```python
from build123d import *

# Parameters (mm, degrees)
BASENUTSKE_R       = 4
BASENUT_DEPTH      = 4
SKETCH6_OUTSIDE_W  = 38.384
SKETCH6_OUTSIDE_H  = 36.372
SKETCH6_OUTSIDE_R  = 6.175
CUT_EXTRUDE2_DEPTH = 5
CUT_EXTRUDE2_TAPER = 60


with BuildPart() as part:
    # BaseNutSke → BaseNut (new body)
    with BuildSketch(Plane.XY):
        Polygon((3.75277675, -6.5), (-3.75277675, -6.5), (-7.505553499, 0), (-3.75277675, 6.5), (3.75277675, 6.5), (7.505553499, 0), align=None)
        Circle(BASENUTSKE_R, mode=Mode.SUBTRACT)
    extrude(amount=-BASENUT_DEPTH)

    # Sketch6 outside → Cut-Extrude2 (cut, through all)
    with BuildSketch(Plane(origin=(0, 0, -4), x_dir=(-1, 0, 0), z_dir=(0, 0, -1))):
        Rectangle(SKETCH6_OUTSIDE_W, SKETCH6_OUTSIDE_H)
        Circle(SKETCH6_OUTSIDE_R, mode=Mode.SUBTRACT)
    cut_extrude2 = extrude(amount=-CUT_EXTRUDE2_DEPTH, taper=CUT_EXTRUDE2_TAPER, mode=Mode.SUBTRACT)

    # Mirror1: Cut-Extrude2 across plane
    add(cut_extrude2.mirror(Plane(origin=(0, 0, -2), x_dir=(1, 0, 0), z_dir=(0, 0, -1))), mode=Mode.SUBTRACT)


solid = part.part
```
Here's how the part is built. I have some questions about the finished solid (model axes, mm). Give positions to 0.01 mm unless a question says otherwise; leave off trailing zeros. Order: outer loops, then holes, each group sorted by start corner. A loop starts at its lowest first (then second) coordinate and runs counter-clockwise, first axis right, second up. Notation, with made-up numbers: (42.5, 40.5) -> (62.5, 40.5) arc R15 ccw to (62.5, 67.5) -> close; hole circle Ø10 at (-16, 57.25). An arc over 180 degrees is marked (long way). Use CSV: the item, a comma, the result in double quotes. Start each with the question number.
Item 1: Suppose I cut it at C-C (z = -3.6). List the corners of the cut face in (x, y) for me.
Item 2: Thinking about a two-plate mould opening in X: for faces 1 (the flat face through (0, 6.5, -2)), 2 (the flat face through (5.6, 3.3, -2)), 3 (the flat face through (-5.66, 3.2, -1.97)), 4 (the cylindrical face through (-0.867, -3.905, -1.972)), which applies, pulls with the +X half, pulls with the -X half, needs draft (parallel to the pull), parting line crosses it, or undercut?
Item 3: Suppose I cut it at A-A (x = 0). List the corners of the cut face in (y, z) for me (3 decimals).
Item 4: Suppose I cut it at B-B (z = -2.75). List the corners of the cut face in (x, y) for me.
Item 5: If I drill on probe 1 along Y at (x, z) = (0, -0.8); probe 2 along X at (y, z) = (0.25, -1.5); probe 3 along X at (y, z) = (-3, -1.3), over which ranges is the centre line in solid material (lowest first)? Write a range as [from, to].
Item 6: I'm going to push a flat-ended pin straight in: P1, Ø1, axis at y = 4, z = -2, coming from the -X side. Where does the tip first touch, or does it pass through?
Answer block:
1,outline,"(-6.74, -1.33) -> (-4.52, -5.17) arc R6.87 ccw to (-2.22, -6.5) -> (2.22, -6.5) arc R6.87 ccw to (4.52, -5.17) -> (6.74, -1.33) arc R6.87 ccw to (6.74, 1.33) -> (4.52, 5.17) arc R6.87 ccw to (2.22, 6.5) -> (-2.22, 6.5) arc R6.87 ccw to (-4.52, 5.17) -> (-6.74, 1.33) arc R6.87 ccw to start; hole circle Ø8 at (0, 0)"
2,face 1,"needs draft"
2,face 2,"pulls with the +X half"
2,face 3,"pulls with the -X half"
2,face 4,"undercut"
3,outline,"(-6.5, -3.812) -> (-6.175, -4) -> (-4, -4) -> (-4, 0) -> (-6.175, 0) -> (-6.5, -0.188) -> close; (4, -4) -> (6.175, -4) -> (6.5, -3.812) -> (6.5, -0.188) -> (6.175, 0) -> (4, 0) -> close"
4,outline,"(-7.51, 0) -> (-3.75, -6.5) -> (3.75, -6.5) -> (7.51, 0) -> (3.75, 6.5) -> (-3.75, 6.5) -> close; hole circle Ø8 at (0, 0)"
5,probe 1,"y = [-6.5, -4], [4, 6.5]"
5,probe 2,"x = [-7.36, -3.99], [3.99, 7.36]"
5,probe 3,"x = [-5.77, -2.65], [2.65, 5.77]"
6,P1,"stops at x = -5.48"
